For this review, take the finished solid that the model builds, in its own axes (mm). Face numbers are marked on the shaded views. A direction names the side the tool comes from. Coordinates: 2 decimals unless noted, no trailing zeros. Write each loop counter-clockwise with the first axis right and the second up, starting at its lowest first coordinate (ties: lowest second). Pieces come first, ordered by that corner, then holes.
1) To check wall thickness, follow line 1 along Y through (x, z) = (21.75, 0); line 2 along X through (y, z) = (15.75, 0); line 3 along X through (y, z) = (9, 1). State the ranges of each line that lie inside material, in increasing order.
2) We need section A-A on z = 0. Write out the cut boundary in (x, y).
3) Mouldability with a two-part tool opening along X and no side actions: class the marked faces 6, 7 and 8 as pulls with the +X half, pulls with the -X half, needs draft (parallel to the pull), parting line crosses it, or undercut.
4) We need section D-D on y = 10. Write out the cut boundary in (x, z), then the cut area to 3 significant figures.
5) We need section C-C on x = 12.5. Write out the cut boundary in (y, z), then the cut area to 3 significant figures.
6) For the marked faces 1, 2, 3, 4 and 5, list the 3-axis set-ups (+Z, -Z, +X, -X, +Y, -Y) from which the entire face can be reached by the end or side of a thin tool; tool diameter is ignored.
7) Insertion check: P1, Ø6, axis at x = 10.5, z = -8.5, coming from the +Y side; P2, Ø1.8, axis at y = -3.5, z = 3.5, coming from the +X side; P3, Ø1, axis at x = 19.5, y = -2, coming from the -Z side. Each pin has a flat end and moves straight along its axis. Give the tip position at first contact, or say it passes through.
8) We need section B-B on y = 2.5. Write out the cut boundary in (x, z), then the cut area to 3 significant figures.
from build123d import *

# Parameters (mm, degrees)
SKETCH1_W           = 25
SKETCH1_H           = 20
BOSS_EXTRUDE1_DEPTH = 20
CUT_EXTRUDE1_DEPTH  = 18
HOLE1_D             = 7
HOLE1_DEPTH         = 6.5
SKETCH6_W           = 15
SKETCH6_H           = 20
BOSS_EXTRUDE2_DEPTH = 6


with BuildPart() as part:
    # Sketch1 → Boss-Extrude1 (new body, symmetric)
    with BuildSketch(Plane.XY):
        with Locations((12.5, 10)):
            Rectangle(SKETCH1_W, SKETCH1_H)
    extrude(amount=BOSS_EXTRUDE1_DEPTH, both=True)

    # Sketch2 → Cut-Extrude1 (cut)
    with BuildSketch(Plane(origin=(0, 20, 0), x_dir=(1, 0, 0), z_dir=(0, 1, 0))):
        with BuildLine():
            Line((6.5, 7.5), (6.5, -7.5))
            ThreePointArc((6.5, -7.5), (12.5, -13.5), (18.5, -7.5))
            Line((18.5, -7.5), (18.5, 7.5))
            ThreePointArc((18.5, 7.5), (12.5, 13.5), (6.5, 7.5))
        make_face()
    extrude(amount=-CUT_EXTRUDE1_DEPTH, mode=Mode.SUBTRACT)

    # Hole1
    with Locations(Plane(origin=(25, 0, 0), x_dir=(0, 0, -1), z_dir=(1, 0, 0))):
        with Locations((0, 10)):
            Hole(HOLE1_D / 2, depth=HOLE1_DEPTH)

    # Sketch6 → Boss-Extrude2 (add)
    with BuildSketch(Plane(origin=(0, 0, 0), x_dir=(1, 0, 0), z_dir=(0, 1, 0))):
        with Locations((12.5, 0)):
            Rectangle(SKETCH6_W, SKETCH6_H)
    extrude(amount=-BOSS_EXTRUDE2_DEPTH)


solid = part.part
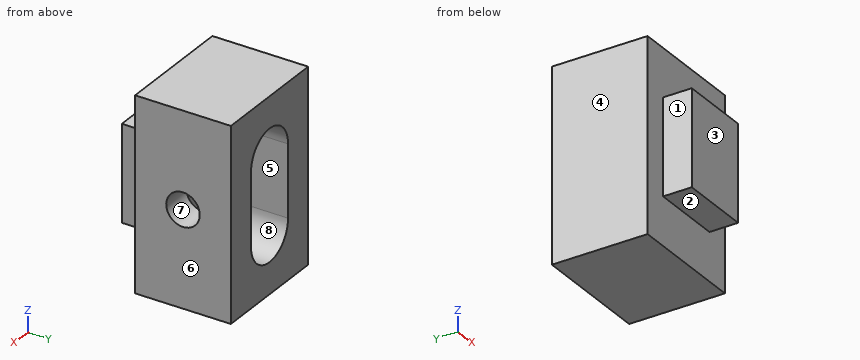
Result:
1. line 1: y = 0 to 6.5, 13.5 to 20
1. line 2: x = 0 to 6.5, 18.5 to 25
1. line 3: x = 0 to 6.5
2. outline: (0, 0) - (5, 0) - (5, -6) - (20, -6) - (20, 0) - (25, 0) - (25, 6.5) - (18.5, 6.5) - (18.5, 2) - (6.5, 2) - (6.5, 20) - (0, 20) - close; (18.5, 13.5) - (25, 13.5) - (25, 20) - (18.5, 20) - close
3. face 6: pulls with the +X half
3. face 7: needs draft
3. face 8: undercut
4. outline: (0, -20) - (25, -20) - (25, -3.5) - (18.5, -3.5) - (18.5, -7.5) arc R6 cw to (6.5, -7.5) - (6.5, 7.5) arc R6 cw to (18.5, 7.5) - (18.5, 3.5) - (25, 3.5) - (25, 20) - (0, 20) - close
4. area: 661 mm2
5. outline: (-6, -10) - (0, -10) - (0, -20) - (20, -20) - (20, -13.5) - (2, -13.5) - (2, 13.5) - (20, 13.5) - (20, 20) - (0, 20) - (0, 10) - (-6, 10) - close
5. area: 434 mm2
6. face 1: +Z, -Z, -X, -Y
6. face 2: -Z, +X, -X, -Y
6. face 3: +Z, -Z, +X, -X, -Y
6. face 4: +Z, -Z, -X, +Y, -Y
6. face 5: +Y
7. P1: stops at y = 2
7. P2: stops at x = 20
7. P3: stops at z = -10
8. outline: (0, -20) - (25, -20) - (25, 20) - (0, 20) - close; hole (6.5, -7.5) arc R6 ccw to (18.5, -7.5) - (18.5, 7.5) arc R6 ccw to (6.5, 7.5) - close
8. area: 707 mm2
